Part model, mm, in its own coordinate system. A direction names the side the tool comes from. Round coordinates to 2 decimals unless told otherwise and drop trailing zeros. Write each loop counter-clockwise with the first axis right and the second up, starting at its lowest first coordinate (ties: lowest second). Pieces come first, ordered by that corner, then holes.
```python
from build123d import *

# Parameters (mm, degrees)
SKETCH1_W           = 13.081
SKETCH1_H           = 32.004
SKETCH1_R           = 5.969
SKETCH1_R_2         = 1.5875
BOSS_EXTRUDE1_DEPTH = 1.5875
SKETCH2_R           = 5.969
BOSS_EXTRUDE2_DEPTH = 8.4455
SKETCH3_W           = 7.493
SKETCH3_H           = 22.86
BOSS_EXTRUDE3_DEPTH = 7.9375
FILLET1_R           = 2.54


with BuildPart() as part:
    # Sketch1 → Boss-Extrude1 (new body)
    # profile 1 of 2: a face of its own
    with BuildSketch(Plane(origin=(0, 0, 0), x_dir=(1, 0, 0), z_dir=(0, 1, 0))):
        Rectangle(SKETCH1_W, SKETCH1_H)
        with Locations((0, 8.89)):
            Circle(SKETCH1_R, mode=Mode.SUBTRACT)
        with Locations(Location((0, 0, 0), (0, 0, 270))):
            Circle(SKETCH1_R_2, mode=Mode.SUBTRACT)
    # profile 2 of 2: a face of its own
    with BuildSketch(Plane(origin=(0, 0, 0), x_dir=(1, 0, 0), z_dir=(0, 1, 0))):
        with Locations((0, 8.89)):
            Circle(SKETCH1_R)
    extrude(amount=BOSS_EXTRUDE1_DEPTH)

    # Sketch2 → Boss-Extrude2 (add)
    with BuildSketch(Plane(origin=(0, 1.5875, 0), x_dir=(1, 0, 0), z_dir=(0, 1, 0))):
        with Locations(Location((0, 8.89, 0), (0, 0, 270))):
            Circle(SKETCH2_R)
    extrude(amount=BOSS_EXTRUDE2_DEPTH)

    # Sketch3 → Boss-Extrude3 (add)
    with BuildSketch(Plane(origin=(0, 1.5875, 0), x_dir=(1, 0, 0), z_dir=(0, 1, 0))):
        with Locations((-0.508, -23.749)):
            Rectangle(SKETCH3_W, SKETCH3_H)
    extrude(amount=BOSS_EXTRUDE3_DEPTH)

    # Fillet1
    fillet1_edges = [part.edges().sort_by_distance(p)[0] for p in [
        (-0.508, 9.525, 12.319),
    ]]
    fillet(fillet1_edges, radius=FILLET1_R)


solid = part.part
```
Q1. Cut at A-A on z = 0. Write the cut outline in (x, y), plus the area to 3 significant figures.
Values follow:
outline: (-6.54, 0) - (-1.59, 0) - (-1.59, 1.59) - (-6.54, 1.59) - close; (1.59, 0) - (6.54, 0) - (6.54, 1.59) - (1.59, 1.59) - close
area: 15.7 mm2
Q2. Mould opens along Z. For faces 1 (the flat face through (-1, 6, 35.179)), 2 (the flat face through (0, 1, -16.002)), 3 (the flat face through (-1, 9.525, 25)), 4 (the flat face through (-1, 4, 12.319)) say: +Z half, -Z half, draft (parallel to the pull), parting line (faces both ways), or undercut.
Values follow:
face 1: +Z half
face 2: -Z half
face 3: draft
face 4: undercut
Q3. Cut at B-B on x = 0. Write the cut outline in (y, z) (1 decimal), plus the area to 3 significant figures.
Values follow:
outline: (0, -16) - (1.6, -16) - (1.6, -14.9) - (10, -14.9) - (10, -2.9) - (1.6, -2.9) - (1.6, -1.6) - (0, -1.6) - close; (0, 1.6) - (1.6, 1.6) - (1.6, 12.3) - (7, 12.3) arc R2.5 ccw to (9.5, 14.9) - (9.5, 35.2) - (1.6, 35.2) - (1.6, 16) - (0, 16) - close
area: 327 mm2
Q4. Which spindle directions (+Z, -Z, +X, -X, +Y, -Y) get a long thin tool onto all of the face, cutting with end or side? Do faces 5 (the cylindrical face through (0.262, 5.751, -14.853)), 6 (the flat face through (0, 1, 16.002)), 7 (the cylindrical face through (-0.46, 8.76, 13.04)). Say none if no direction does.
Values follow:
face 5: +Y
face 6: +Z, +X, -X, -Y
face 7: +X, -X, +Y
Q5. Wall check: L1, parallel to X at y = 1.1, z = 0; L2, parallel to X at y = 5, z = 13; L3, parallel to Z at x = -2.75, y = 8. Give the ranges that are in metal, low to high.
Values follow:
L1: x = -6.54 to -1.59, 1.59 to 6.54
L2: x = -4.25 to 3.24
L3: z = -14.19 to -3.59, 12.53 to 35.18
Q6. Cut at D-D on x = 5.5. Write the cut outline in (y, z), plus the area to 3 significant figures.
Values follow:
outline: (0, -16) - (1.59, -16) - (1.59, -11.21) - (10.03, -11.21) - (10.03, -6.57) - (1.59, -6.57) - (1.59, 16) - (0, 16) - close
area: 90.0 mm2
Q7. Cut at C-C on y = 5.25. Write the cut outline in (x, z), plus the area to 3 significant figures.
Values follow:
outline: circle Ø11.94 at (0, -8.89); (-4.25, 12.32) - (3.24, 12.32) - (3.24, 35.18) - (-4.25, 35.18) - close
area: 283 mm2
Q8. Drop flat-ended pins along their axis: pin 1 (3.5 mm diameter, centred on x = 1, z = 24.5, fed in from +Y) (3 decimals); pin 2 (2.5 mm diameter, centred on y = 4.5, z = 24.5, fed in from +X); pin 3 (5 mm diameter, centred on x = 0, z = -2.5, fed in from -Y); pin 4 (0.8 mm diameter, centred on x = -1, y = 1, fed in from +Z). Give the stop position or say it passes through.
Values follow:
pin 1: stops at y = 9.525
pin 2: stops at x = 3.24
pin 3: stops at y = 0
pin 4: stops at z = 16
